```python
from build123d import *

# Parameters (mm, degrees)
F1_DEPTH = 6.35


with BuildPart() as f1:
    # F0 (on Front) → F1 (new body)
    with BuildSketch(Plane.XZ):
        Polygon((52.898277, 196.296548), (46.718386, 197.756498), (40.538496, 199.216447), (-5.834989, 2.919899), (-5.834989, 1.378469), (0, 0), (6.524792, -1.54143), (6.524792, 0), align=None)
        Polygon((0, 0), (-5.834989, 1.378469), (-5.834989, -111.380101), (6.524792, -111.380101), (6.524792, -1.54143), align=None)
    extrude(amount=F1_DEPTH)


solid = f1.part
```
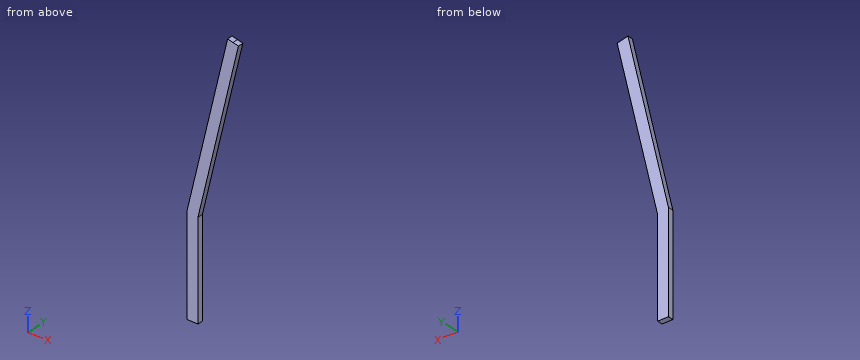
Here's how the part is built. I have some questions about the finished solid (model axes, mm). Coordinates: 2 decimals unless noted, no trailing zeros. Write each loop counter-clockwise with the first axis right and the second up, starting at its lowest first coordinate (ties: lowest second). Pieces come first, ordered by that corner, then holes. Notation, with made-up numbers: M 17.5,27 L 35.5,27 A16 ccw 35.5,35 Z; hole C 89.25,-10 d10. An arc over 180 degrees is marked long. Answer as CSV lines item,"result". Start each with the question number.
Q1. Will these pins go through, and if not, where does the flat tip stop? pin 1 Ø1.5 at (y, z) = (-3.5, 7) entering from -X; pin 2 Ø2 at (y, z) = (-1.5, 59) entering from +X.
Q2. Suppose I cut it at B-B, the plane z = -47. List the corners of the cut face in (x, y) for me.
Q3. Suppose I cut it at A-A, the plane y = -1.75. List the corners of the cut face in (x, z) for me, then the cut area to 3 significant figures.
Q4. Suppose I cut it at C-C, the plane x = 1.5. List the corners of the cut face in (y, z) for me.
Q5. I need wall thicknesses on probe 1 along X at (y, z) = (-2.5, -13); probe 2 along X at (y, z) = (-5.5, 24.5). Which ranges of each line are inside material? Lowest first, please. Write a range as [from, to].
Entries:
1,pin 1,"stops at x = -5.05"
1,pin 2,"stops at x = 20.7"
2,outline,"M -5.83,-6.35 L 6.52,-6.35 L 6.52,0 L -5.83,0 Z"
3,outline,"M -5.83,-111.38 L 6.52,-111.38 L 6.52,0 L 52.9,196.3 L 46.72,197.76 L 40.54,199.22 L -5.83,2.92 Z"
3,area,"3,960 mm²"
4,outline,"M -6.35,-111.38 L 0,-111.38 L 0,33.97 L -6.35,33.97 Z"
5,probe 1,"x = [-5.83, 6.52]"
5,probe 2,"x = [-0.74, 12.31]"
